Could you check a few things on this model? Use its own coordinates, in mm. Face numbers are marked on the shaded views. A direction names the side the tool comes from. Give positions to 0.01 mm unless a question says otherwise; leave off trailing zeros. Loops run counter-clockwise (first coordinate to the right, second up) from the corner with the lowest first, then second, coordinate; pieces in that order, holes last. Notation, with made-up numbers: (27, 70.25) -> (40, 70.25) arc R8 cw to (40, 82.25) -> close; hole circle Ø1 at (-32.5, 21). An arc over 180 degrees is marked (long way). Put each result on its own line as item: value.
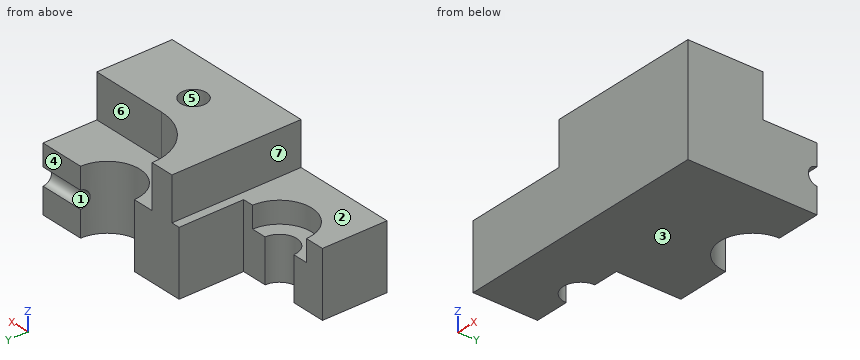
```python
from build123d import *

# Parameters (mm, degrees)
F0_W           = 60
F0_H           = 60
F1_DEPTH       = 25
F2_W           = 24
F2_H           = 60
F3_DEPTH       = 10
F5_D           = 8
F5_CBORE_D     = 15
F5_CBORE_DEPTH = 5
F6_R           = 7.5
F7_DEPTH       = 15
F9_D           = 6
F9_DEPTH       = 15
F9_TIP         = 1.8025818571
F10_R          = 2
F11_DEPTH      = 10.7725839526
F14_DEPTH      = 25


with BuildPart() as f1:
    # F0 (on Top) → F1 (new body)
    with BuildSketch(Plane.XY):
        Rectangle(F0_W, F0_H)
    extrude(amount=F1_DEPTH)

    # F2 (on face) → F3 (cut)
    with BuildSketch(Plane.XY.offset(25)):
        with Locations((-18, 0)):
            Rectangle(F2_W, F2_H)
        with BuildLine():
            Line((30, -12.5), (30, 12.5))
            Line((30, 12.5), (12, 12.5))
            ThreePointArc((12, 12.5), (-0.5, 0), (12, -12.5))
            Line((12, -12.5), (30, -12.5))
        make_face()
    extrude(amount=-F3_DEPTH, mode=Mode.SUBTRACT)

    # F5 (through all)
    with Locations(Plane.XY.offset(15)):
        with Locations((-18, 15), (-18, -15)):
            CounterBoreHole(F5_D / 2, F5_CBORE_D / 2, F5_CBORE_DEPTH)

    # F6 (on face) → F7 (cut, through all)
    with BuildSketch(Plane.XY.offset(15)):
        with Locations((12, 0)):
            Circle(F6_R)
    extrude(amount=-F7_DEPTH, mode=Mode.SUBTRACT)

    # F9
    with Locations(Plane.XY.offset(25)):
        with Locations((12, 20), (12, -20)):
            Hole(F9_D / 2, depth=F9_DEPTH)
            with Locations((0, 0, -(F9_DEPTH + F9_TIP / 2))):  # 118° drill point
                Cone(0, F9_D / 2, F9_TIP, mode=Mode.SUBTRACT)

    # F10 (on face) → F11 (cut, through all)
    with BuildSketch(Plane.YZ.offset(30)):
        with Locations((0, 8)):
            Circle(F10_R)
    extrude(amount=-F11_DEPTH, mode=Mode.SUBTRACT)

    # F13 (on Top) → F14 (cut, through all)
    with BuildSketch(Plane.XY):
        Polygon((-8, 0), (30, 0), (30, 30), (-30, 30), (-30, -15), (-8, -15), align=None)
    extrude(amount=F14_DEPTH, mode=Mode.SUBTRACT)


solid = f1.part
```
1. If we section it at B-B (x = 25): List the corners of the cut face in (y, z) for me.
Recorded:
outline: (-30, 0) -> (0, 0) -> (0, 6) arc R2 cw to (0, 10) -> (0, 15) -> (-12.5, 15) -> (-12.5, 25) -> (-30, 25) -> close
2. Thinking about a two-plate mould opening in Z: for the marked faces 1, 2, 3 and 4, which applies, pulls with the +Z half, pulls with the -Z half, needs draft (parallel to the pull), parting line crosses it, or undercut?
Recorded:
face 1: undercut
face 2: pulls with the +Z half
face 3: pulls with the -Z half
face 4: needs draft
3. If we section it at A-A (z = 12.75): List the corners of the cut face in (x, y) for me, then the cut area to 3 significant figures.
Recorded:
outline: (-30, -30) -> (30, -30) -> (30, 0) -> (19.5, 0) arc R7.5 cw to (4.5, 0) -> (-8, 0) -> (-8, -15) -> (-10.5, -15) arc R7.5 cw to (-25.5, -15) -> (-30, -15) -> close; hole circle Ø6 at (12, -20)
area: 1,270 mm^2
4. I need wall thicknesses on line 1 (Y direction, x = 12, z = 16.25); line 2 (X direction, y = -18, z = 10.75); line 3 (X direction, y = -20, z = 22). Which ranges of each line are inside material? Lowest first, please.
Recorded:
line 1: y = -30 to -23, -17 to -12.5
line 2: x = -30 to -24.87, -11.13 to 9.76, 14.24 to 30
line 3: x = -6 to 9, 15 to 30
5. For the marked faces 5, 6 and 7, which set-ups out of +Z, -Z, +X, -X, +Y, -Y let a thin tool reach every point of the face, with its end or its side?
Recorded:
face 5: +Z
face 6: +Z, +X, +Y
face 7: +Z, -X, +Y, -Y
6. If we section it at D-D (x = 3): List the corners of the cut face in (y, z) for me, then the cut area to 3 significant figures.
Recorded:
outline: (-30, 0) -> (0, 0) -> (0, 15) -> (-8.67, 15) -> (-8.67, 25) -> (-30, 25) -> close
area: 663 mm^2
7. I'm going to push flat-ended pins straight in: pin 1 (4 mm diameter, centred on x = 22, y = -4.5, fed in from +Z); pin 2 (3 mm diameter, centred on y = -9, z = 18.5, fed in from -X); pin 3 (5 mm diameter, centred on x = 18, z = 19, fed in from +Y). Where does each tip first touch, or does it pass through?
Recorded:
pin 1: stops at z = 15
pin 2: stops at x = -6
pin 3: stops at y = -12.5
8. If we section it at C-C (y = -13.5): List the corners of the cut face in (x, z) for me, then the cut area to 3 significant figures.
Recorded:
outline: (-8, 0) -> (30, 0) -> (30, 25) -> (-6, 25) -> (-6, 15) -> (-8, 15) -> close
area: 930 mm^2
